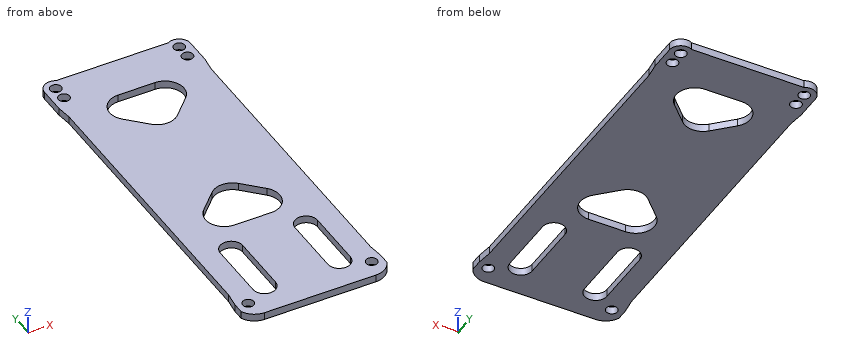
```python
from build123d import *

# Parameters (mm, degrees)
PAD_DEPTH    = 2
SKETCH001_R  = 1.5
POCKET_DEPTH = 2.001


with BuildPart() as part:
    # Sketch → Pad (new body)
    with BuildSketch(Plane.XY):
        with BuildLine():
            Line((-14.886358, -61), (14.886358, -61))
            ThreePointArc((14.886358, -61), (17.657976, -60.161506), (19.5, -57.927254))
            Line((19.5, -54.927254), (19.5, -57.927254))
            Line((19, -50.958627), (19.5, -54.927254))
            Line((19, 26.531373), (19, -50.958627))
            Line((19, 26.531373), (19.5, 30.5))
            Line((19.5, 30.5), (19.5, 37.5))
            ThreePointArc((19.5, 37.5), (18, 40.098076), (15, 40.098076))
            Line((-15, 40.098076), (15, 40.098076))
            ThreePointArc((-15, 40.098076), (-18, 40.098076), (-19.5, 37.5))
            Line((-19.5, 30.5), (-19.5, 37.5))
            Line((-19, 26.531373), (-19.5, 30.5))
            Line((-19, 26.531373), (-19, -50.958627))
            Line((-19, -50.958627), (-19.5, -54.927254))
            Line((-19.5, -54.927254), (-19.5, -57.927254))
            ThreePointArc((-19.5, -57.927254), (-17.657976, -60.161506), (-14.886358, -61))
        make_face()
        with BuildLine():
            ThreePointArc((-7, -36), (-10, -33), (-13, -36))
            Line((-13, -36), (-13, -52))
            ThreePointArc((-13, -52), (-10, -55), (-7, -52))
            Line((-7, -36), (-7, -52))
        make_face(mode=Mode.SUBTRACT)
        with BuildLine():
            ThreePointArc((13, -36), (10, -33), (7, -36))
            Line((7, -36), (7, -52))
            ThreePointArc((7, -52), (10, -55), (13, -52))
            Line((13, -36), (13, -52))
        make_face(mode=Mode.SUBTRACT)
        with BuildLine():
            Line((-8.450534, 19.749437), (-3.535534, 14.834437))
            ThreePointArc((-3.535534, 14.834437), (0, 13.369971), (3.535534, 14.834437))
            Line((3.535534, 14.834437), (8.450534, 19.749437))
            ThreePointArc((8.450534, 19.749437), (9.534398, 25.198388), (4.915, 28.284971))
            Line((4.915, 28.284971), (-4.915, 28.284971))
            ThreePointArc((-4.915, 28.284971), (-9.534398, 25.198388), (-8.450534, 19.749437))
        make_face(mode=Mode.SUBTRACT)
        with BuildLine():
            Line((3.535534, -14.834437), (8.450534, -19.749437))
            ThreePointArc((4.915, -28.284971), (9.534398, -25.198388), (8.450534, -19.749437))
            Line((4.915, -28.284971), (-4.915, -28.284971))
            ThreePointArc((-8.450534, -19.749437), (-9.534398, -25.198388), (-4.915, -28.284971))
            Line((-8.450534, -19.749437), (-3.535534, -14.834437))
            ThreePointArc((3.535534, -14.834437), (0, -13.369971), (-3.535534, -14.834437))
        make_face(mode=Mode.SUBTRACT)
    extrude(amount=PAD_DEPTH)

    # Sketch001 → Pocket (cut, through all)
    with BuildSketch(Plane.XY.offset(2)):
        with Locations((-16.5, 33.5)):
            Circle(SKETCH001_R)
        with Locations((16.5, 33.5)):
            Circle(SKETCH001_R)
        with Locations((16.5, -56)):
            Circle(SKETCH001_R)
        with Locations((-16.5, -56)):
            Circle(SKETCH001_R)
        with Locations((16.5, 37.5)):
            Circle(SKETCH001_R)
        with Locations((-16.5, 37.5)):
            Circle(SKETCH001_R)
    extrude(amount=-POCKET_DEPTH, mode=Mode.SUBTRACT)


solid = part.part
```
CAD build for the part. Positions are in the model's coordinates, mm. Round coordinates to 2 decimals unless told otherwise and drop trailing zeros. Order: outer loops, then holes, each group sorted by start corner. A loop starts at its lowest first (then second) coordinate and runs counter-clockwise, first axis right, second up.
Item 1: Saw through at D-D on y = -16. Write the cut outline in (x, z).
Item 2: Pin check, flat tips, straight feed: pin 1 (0.6 mm diameter, centred on y = -41, z = 1.5, fed in from -X); pin 2 (2.5 mm diameter, centred on x = 16.5, y = -56, fed in from +Z); pin 3 (1 mm diameter, centred on x = -4, z = 1.5, fed in from +Y). Stop position of each tip, or through.
Item 3: Saw through at C-C on x = 16.5. Write the cut outline in (y, z).
Item 4: Probe line 1 along Y through (x, z) = (16.5, 1.4); line 2 along Y through (x, z) = (8, 1.35); line 3 along Y through (x, z) = (-1, 0.5). List the from-to ranges inside material, lowest first.
Item 5: Saw through at A-A on y = -56. Write the cut outline in (x, z), then the cut area to 3 significant figures.
Item 6: Saw through at B-B on x = -11. Write the cut outline in (y, z), then the cut area to 3 significant figures.
Reported:
1. outline: (-19, 0) - (-4.7, 0) - (-4.7, 2) - (-19, 2) - close; (4.7, 0) - (19, 0) - (19, 2) - (4.7, 2) - close
2. pin 1: stops at x = -19
2. pin 2: passes through
2. pin 3: stops at y = 40.1
3. outline: (-60.73, 0) - (-57.5, 0) - (-57.5, 2) - (-60.73, 2) - close; (-54.5, 0) - (32, 0) - (32, 2) - (-54.5, 2) - close; (35, 0) - (36, 0) - (36, 2) - (35, 2) - close; (39, 0) - (40.5, 0) - (40.5, 2) - (39, 2) - close
4. line 1: y = -60.73 to -57.5, -54.5 to 32, 35 to 36, 39 to 40.5
4. line 2: y = -61 to -54.24, -33.76 to -27.22, -19.3 to 19.3, 27.22 to 40.1
4. line 3: y = -61 to -28.28, -13.47 to 13.47, 28.28 to 40.1
5. outline: (-19.5, 0) - (-18, 0) - (-18, 2) - (-19.5, 2) - close; (-15, 0) - (15, 0) - (15, 2) - (-15, 2) - close; (18, 0) - (19.5, 0) - (19.5, 2) - (18, 2) - close
5. area: 66.0 mm2
6. outline: (-61, 0) - (-54.83, 0) - (-54.83, 2) - (-61, 2) - close; (-33.17, 0) - (40.1, 0) - (40.1, 2) - (-33.17, 2) - close
6. area: 159 mm2
